from build123d import *

# Parameters (mm, degrees)
SKETCH2_R           = 0.25
BOSS_EXTRUDE1_DEPTH = 4


with BuildPart() as part:
    # Sketch1 → Revolve1 (revolve)
    with BuildSketch(Plane(origin=(0, 0, 0), x_dir=(0, 0, -1), z_dir=(1, 0, 0))):
        with BuildLine():
            Line((-2.5, 6.2), (-2.5, 1))
            Line((-2.5, 1), (-2.9, 1))
            Line((-2.9, 1), (-2.9, 0))
            Line((-2.9, 0), (0, 0))
            Line((0, 0), (0, 8.7))
            ThreePointArc((0, 8.7), (-1.767766953, 7.967766953), (-2.5, 6.2))
        make_face()
    revolve(axis=Axis((0, 16.477597325, 0), (0, -1, 0)))

    # Sketch2 → Boss-Extrude1 (add)
    with BuildSketch(Plane.XZ):
        with Locations(Location((-1.95, 0, 0), (0, 0, 270))):
            Circle(SKETCH2_R)
        with Locations(Location((-0.65, 0, 0), (0, 0, 270))):
            Circle(SKETCH2_R)
        with Locations(Location((0.65, 0, 0), (0, 0, 90))):
            Circle(SKETCH2_R)
        with Locations(Location((1.95, 0, 0), (0, 0, 90))):
            Circle(SKETCH2_R)
    extrude(amount=BOSS_EXTRUDE1_DEPTH)


solid = part.part
Input: part model. Units: mm. Frame: model coordinates. A direction names the side the tool comes from. Coordinates: 2 decimals unless noted, no trailing zeros. Loops run counter-clockwise (first coordinate to the right, second up) from the corner with the lowest first, then second, coordinate; pieces in that order, holes last. Notation, with made-up numbers: (-35, -27.5) -> (0, -27.5) arc R20 ccw to (0, 7.5) -> close; hole circle Ø3 at (0.5, -29). An arc over 180 degrees is marked (long way). Write each question's results on one line, items separated by ' | '. Start each with the question number.
Q1. Section D-D, the plane y = 5.25. Return the cut outline in (x, z), plus the area to 3 significant figures.
Q2. Section A-A, the plane z = -2. Return the cut outline in (x, y).
Q3. Pin query (flat end, axial travel): pin 1 (1.5 mm diameter, centred on y = 5.5, z = 2, fed in from -X); pin 2 (1.7 mm diameter, centred on x = 1, z = -0.5, fed in from +Y); pin 3 (3 mm diameter, centred on y = 6.5, z = -2, fed in from +X). Return the tip coordinate at first contact, or that it passes through.
Q4. Section C-C, the plane y = -1.5. Return the cut outline in (x, z), plus the area to 3 significant figures.
Q5. Ray query, line 1 (Z direction, x = -2.3, y = 4); line 2 (Y direction, x = -0.3, z = 1.3); line 3 (X direction, y = 0.25, z = -0.9). Return the intervals inside material, ascending. Write a range as from..to.
Q6. Reachability of faces 1 (the cylindrical face through (-0.1, 0.5, -2.9)), 2 (the cylindrical face through (2.44, 3.56, -0.54)) from +Z, -Z, +X, -X, +Y, -Y: full face, straight path, thin tool, end or side. Return the list, or none.
Q7. Section B-B, the plane x = 0. Return the cut outline in (y, z).
Found:
1) outline: circle Ø5 at (0, 0) | area: 19.6 mm2
2) outline: (-2.1, 0) -> (2.1, 0) -> (2.1, 1) -> (1.5, 1) -> (1.5, 6.2) arc R1.5 ccw to (-1.5, 6.2) -> (-1.5, 1) -> (-2.1, 1) -> close
3) pin 1: x = -2.17 | pin 2: y = 8.69 | pin 3: x = 2.44
4) outline: circle Ø0.5 at (-1.95, 0); circle Ø0.5 at (-0.65, 0); circle Ø0.5 at (0.65, 0); circle Ø0.5 at (1.95, 0) | area: 0.785 mm2
5) line 1: -0.98..0.98 | line 2: 0..8.31 | line 3: -2.76..2.76
6) face 1: +Y, -Y | face 2: +Y
7) outline: (0, -2.9) -> (1, -2.9) -> (1, -2.5) -> (6.2, -2.5) arc R2.5 ccw to (6.2, 2.5) -> (1, 2.5) -> (1, 2.9) -> (0, 2.9) -> close
